CAD build for the part. Positions are in the model's coordinates, mm. Round coordinates to 2 decimals unless told otherwise and drop trailing zeros. Loops run counter-clockwise (first coordinate to the right, second up) from the corner with the lowest first, then second, coordinate; pieces in that order, holes last.
from build123d import *

# Parameters (mm, degrees)
F0_W     = 30
F0_H     = 30
F0_R     = 2.25
F1_DEPTH = 5
F2_SIZE  = 1.5


with BuildPart() as f1:
    # F0 (on Top) → F1 (new body)
    with BuildSketch(Plane.XY):
        Rectangle(F0_W, F0_H)
        with Locations((-10, -10)):
            Circle(F0_R, mode=Mode.SUBTRACT)
        with Locations((10, -10)):
            Circle(F0_R, mode=Mode.SUBTRACT)
        with Locations((-10, 10)):
            Circle(F0_R, mode=Mode.SUBTRACT)
        with Locations((10, 10)):
            Circle(F0_R, mode=Mode.SUBTRACT)
    extrude(amount=F1_DEPTH)

    # F2
    f2_edges = [f1.edges().sort_by_distance(p)[0] for p in [
        (-12.25, -10, 5),
        (-12.25, 10, 5),
        (7.75, -10, 5),
        (7.75, 10, 5),
    ]]
    chamfer(f2_edges, length=F2_SIZE)


solid = f1.part
Item 1: Cut at D-D (z = 4.5). List the corners of the cut face in (x, y).
Verdict:
outline: (-15, -15) - (15, -15) - (15, 15) - (-15, 15) - close; hole circle Ø6.5 at (-10, -10); hole circle Ø6.5 at (-10, 10); hole circle Ø6.5 at (10, -10); hole circle Ø6.5 at (10, 10)
Item 2: Cut at A-A (z = 1.3). List the corners of the cut face in (x, y), plus the area to 3 significant figures.
Verdict:
outline: (-15, -15) - (15, -15) - (15, 15) - (-15, 15) - close; hole circle Ø4.5 at (-10, -10); hole circle Ø4.5 at (-10, 10); hole circle Ø4.5 at (10, -10); hole circle Ø4.5 at (10, 10)
area: 836 mm2
Item 3: Cut at B-B (y = 10). List the corners of the cut face in (x, z).
Verdict:
outline: (-15, 0) - (-12.25, 0) - (-12.25, 3.5) - (-13.75, 5) - (-15, 5) - close; (-7.75, 0) - (7.75, 0) - (7.75, 3.5) - (6.25, 5) - (-6.25, 5) - (-7.75, 3.5) - close; (12.25, 0) - (15, 0) - (15, 5) - (13.75, 5) - (12.25, 3.5) - close
Item 4: Mould opens along Y. For faces 1 (the flat face through (0, 15, 2)), 2 (the flat face through (0, 0, 5)), 3 (the cylindrical face through (8.34, -8.48, 1.73)) say: released by +Y, released by -Y, zero draft, split by the parting line, or undercut.
Verdict:
face 1: released by +Y
face 2: zero draft
face 3: undercut
Item 5: Wall check: L1, parallel to Y at x = 10, z = 1.5; L2, parallel to X at y = -8.5, z = 4.6; L3, parallel to Y at x = 8, z = 3.9. Give the ranges that are in metal, low to high.
Verdict:
L1: y = -15 to -12.25, -7.75 to 7.75, 12.25 to 15
L2: x = -15 to -13, -7 to 7, 13 to 15
L3: y = -15 to -11.74, -8.26 to 8.26, 11.74 to 15
Item 6: Flat gauge pin, fed straight in: P1, Ø6, axis at x = 10, y = -10, coming from the +Z side. Where does the tip first touch, or does it go through?
Verdict:
P1: stops at z = 4.25
